from build123d import *

# Parameters (mm, degrees)
SKETCH_2_W               = 140.3
SKETCH_2_H               = 48.7
EXTRUDE_1_DEPTH          = 4
SKETCH_3_W               = 140.3
SKETCH_3_H               = 48.7
SKETCH_3_R               = 1.6
SKETCH_3_W_2             = 129
SKETCH_3_H_2             = 44.9
CUT_EXTRUDE_1_DEPTH      = 2
SKETCH_6_W               = 54
SKETCH_6_H               = 44.9
SKETCH_6_W_2             = 3
SKETCH_6_W_3             = 13
SKETCH_6_H_2             = 13
SKETCH_6_W_4             = 10
SKETCH_6_H_3             = 16
SKETCH_6_R               = 1.6
CUT_EXTRUDE_2_DEPTH      = 149.565743023
CUT_EXTRUDE_3_DEPTH      = 149.565743023
CUT_EXTRUDE_3_DEPTH_BACK = 10
SKETCH_7_W               = 6.5
SKETCH_7_H               = 16


with BuildPart() as part:
    # 草图2 → 凸台-拉伸1 (new body)
    with BuildSketch(Plane.XY):
        with Locations((70.15, 24.35)):
            Rectangle(SKETCH_2_W, SKETCH_2_H)
    extrude(amount=EXTRUDE_1_DEPTH)

    # 草图3 → 切除-拉伸1 (cut)
    with BuildSketch(Plane.XY.offset(4)):
        with Locations((70.15, 24.35)):
            Rectangle(SKETCH_3_W, SKETCH_3_H)
        with Locations((138.1, 1.8)):
            Circle(SKETCH_3_R, mode=Mode.SUBTRACT)
        with Locations((138.1, 44.7)):
            Circle(SKETCH_3_R, mode=Mode.SUBTRACT)
        with Locations((2.5, 1.8)):
            Circle(SKETCH_3_R, mode=Mode.SUBTRACT)
        with Locations((2.5, 44.7)):
            Circle(SKETCH_3_R, mode=Mode.SUBTRACT)
        with Locations((70.8, 24.25)):
            Rectangle(SKETCH_3_W_2, SKETCH_3_H_2, mode=Mode.SUBTRACT)
    extrude(amount=-CUT_EXTRUDE_1_DEPTH, mode=Mode.SUBTRACT)

    # 草图6 → 切除-拉伸2 (cut, through all)
    with BuildSketch(Plane.XY.offset(4)):
        with Locations((108.3, 24.25)):
            Rectangle(SKETCH_6_W, SKETCH_6_H)
        with Locations((72.8, 24.25)):
            Rectangle(SKETCH_6_W_2, SKETCH_6_H)
        with Locations((42.8, 40.2)):
            Rectangle(SKETCH_6_W_3, SKETCH_6_H_2)
        with Locations((21.3, 15.7)):
            Rectangle(SKETCH_6_W_4, SKETCH_6_H_3)
        with Locations((2.5, 44.7)):
            Circle(SKETCH_6_R)
        with Locations((2.5, 1.8)):
            Circle(SKETCH_6_R)
        with Locations((138.1, 44.7)):
            Circle(SKETCH_6_R)
        with Locations((138.1, 1.8)):
            Circle(SKETCH_6_R)
    extrude(amount=-CUT_EXTRUDE_2_DEPTH, mode=Mode.SUBTRACT)

    # 草图7 → 切除-拉伸3 (cut, two sides: drawn at the far end of the back side and taken through both)
    with BuildSketch(Plane(origin=(0, 0, 0), x_dir=(-1, 0, 0), z_dir=(0, 0, -1)).offset(-CUT_EXTRUDE_3_DEPTH_BACK)):
        with Locations((-13.05, 15.7)):
            Rectangle(SKETCH_7_W, SKETCH_7_H)
    extrude(amount=CUT_EXTRUDE_3_DEPTH + CUT_EXTRUDE_3_DEPTH_BACK, mode=Mode.SUBTRACT)


solid = part.part
Could you check a few things on this model? Use its own coordinates, in mm. A direction names the side the tool comes from. Give positions to 0.01 mm unless a question says otherwise; leave off trailing zeros. Order: outer loops, then holes, each group sorted by start corner. A loop starts at its lowest first (then second) coordinate and runs counter-clockwise, first axis right, second up.
1. I need wall thicknesses on L1, parallel to Y at x = 2.5, z = 1; L2, parallel to X at y = 45, z = 3.4; L3, parallel to X at y = 22.5, z = 0.55. Which ranges of each line are inside material? Lowest first, please.
2. We'd pull the mould along X, two halves only. Please class faces 3 (the flat face through (36.3, 40, 2)), 4 (the flat face through (38, 25, 0)), 5 (the flat face through (43, 33.7, 2)): pulls with the +X half, pulls with the -X half, needs draft (parallel to the pull), parting line crosses it, or undercut.
3. Will these pins go through, and if not, where does the flat tip stop? P1, Ø5, axis at x = 2.5, y = 1.8, coming from the +Z side; P2, Ø1, axis at x = 76.5, z = 3, coming from the -Y side; P3, Ø2, axis at x = 20, z = 2, coming from the -Y side; P4, Ø1, axis at x = 16.5, z = 3.5, coming from the +Y side.
4. Suppose I cut it at C-C (z = 1.25). Give the number of separate pieces and of enclosed holes in the cut face, plus the area to 3 significant figures.
5. Suppose I cut it at B-B (y = 30). List the corners of the cut face in (x, z) for me.
6. Suppose I cut it at D-D (x = 87). List the corners of the cut face in (y, z) for me, plus the area to 3 significant figures.
7. For faces 1 (the flat face through (78, 25, 4)), 2 (the flat face through (18, 7.7, 2)), which set-ups out of +Z, -Z, +X, -X, +Y, -Y let a thin tool reach every point of the face, with its end or its side?
8. Suppose I cut it at A-A (x = 2.5). List the corners of the cut face in (y, z) for me, plus the area to 3 significant figures.
Solved:
1. L1: y = 0 to 0.2, 3.4 to 43.1, 46.3 to 48.7
1. L2: x = 6.3 to 36.3, 49.3 to 71.3, 74.3 to 81.3
1. L3: x = 0 to 9.8, 26.3 to 71.3, 74.3 to 81.3, 135.3 to 140.3
2. face 3: undercut
2. face 4: needs draft
2. face 5: undercut
3. P1: stops at z = 2
3. P2: stops at y = 1.8
3. P3: stops at y = 0
3. P4: stops at y = 46.7
4. separate pieces: 1
4. enclosed holes: 8
4. area: 3,810 mm2
5. outline: (0, 0) - (71.3, 0) - (71.3, 4) - (6.3, 4) - (6.3, 2) - (0, 2) - close; (74.3, 0) - (81.3, 0) - (81.3, 4) - (74.3, 4) - close; (135.3, 0) - (140.3, 0) - (140.3, 2) - (135.3, 2) - close
6. outline: (0, 0) - (1.8, 0) - (1.8, 2) - (0, 2) - close; (46.7, 0) - (48.7, 0) - (48.7, 2) - (46.7, 2) - close
6. area: 7.60 mm2
7. face 1: +Z, +X, -X, +Y, -Y
7. face 2: +Z, -Z
8. outline: (0, 0) - (0.2, 0) - (0.2, 2) - (0, 2) - close; (3.4, 0) - (43.1, 0) - (43.1, 2) - (3.4, 2) - close; (46.3, 0) - (48.7, 0) - (48.7, 2) - (46.3, 2) - close
8. area: 84.6 mm2
